Could you check a few things on this model? Use its own coordinates, in mm. A direction names the side the tool comes from. Give positions to 0.01 mm unless a question says otherwise; leave off trailing zeros. Order: outer loops, then holes, each group sorted by start corner. A loop starts at its lowest first (then second) coordinate and runs counter-clockwise, first axis right, second up. Notation, with made-up numbers: (89.25, -28.75) -> (134.25, -28.75) arc R13 ccw to (134.25, -14.75) -> close; hole circle Ø1 at (47.5, 83). An arc over 180 degrees is marked (long way). Write each question's results on one line, items separated by ' | '.
```python
from build123d import *

# Parameters (mm, degrees)
F1_DEPTH = 15


with BuildPart() as f1:
    # F0 (on Top) → F1 (new body)
    with BuildSketch(Plane.XY):
        Polygon((-70.779354, 10.755781), (-72.929354, 10.755781), (-72.929354, -4.244219), (-72.029354, -4.244219), (-68.829354, -4.244219), (-67.929354, -4.244219), (-67.929354, 10.755781), (-70.079354, 10.755781), align=None)
        Polygon((-71.429354, 14.255781), (-70.779354, 10.755781), (-70.079354, 10.755781), (-69.429354, 14.255781), align=None)
        Polygon((-72.029354, -4.244219), (-72.929354, -4.244219), (-72.929354, -7.944219), (-71.429354, -7.944219), align=None)
        Polygon((-67.929354, -4.244219), (-68.829354, -4.244219), (-69.429354, -7.944219), (-67.929354, -7.944219), align=None)
    extrude(amount=F1_DEPTH)


solid = f1.part
```
Q1. Suppose I cut it at B-B on y = -4.5. Please give me the cut outline in (x, z).
Here are the results:
outline: (-72.93, 0) -> (-71.99, 0) -> (-71.99, 15) -> (-72.93, 15) -> close; (-68.87, 0) -> (-67.93, 0) -> (-67.93, 15) -> (-68.87, 15) -> close
Q2. Thinking about a two-plate mould opening in X: for faces 6 (the flat face through (-71.11, 12.53, 7.4)), 7 (the flat face through (-69.125, -6.068, 7.395)), 8 (the flat face through (-69, 10.756, 7)), which applies, +X half, -X half, draft (parallel to the pull), parting line (faces both ways), or undercut?
Here are the results:
face 6: -X half | face 7: undercut | face 8: draft
Q3. Suppose I cut it at C-C on z = 13.5. Please give me the cut outline in (x, y).
Here are the results:
outline: (-72.93, -7.94) -> (-71.43, -7.94) -> (-72.03, -4.24) -> (-68.83, -4.24) -> (-69.43, -7.94) -> (-67.93, -7.94) -> (-67.93, 10.76) -> (-70.08, 10.76) -> (-69.43, 14.26) -> (-71.43, 14.26) -> (-70.78, 10.76) -> (-72.93, 10.76) -> close
Q4. Suppose I cut it at A-A on x = -69.05. Please give me the cut outline in (y, z).
Here are the results:
outline: (-7.94, 0) -> (-5.6, 0) -> (-5.6, 15) -> (-7.94, 15) -> close; (-4.24, 0) -> (10.76, 0) -> (10.76, 15) -> (-4.24, 15) -> close
Q5. I need wall thicknesses on line 1 along Y through (x, z) = (-68.7, 14); line 2 along Y through (x, z) = (-70.5, 2.25); line 3 along X through (y, z) = (-4.75, 4.25). Which ranges of each line are inside material? Lowest first, please.
Here are the results:
line 1: y = -7.94 to 10.76 | line 2: y = -4.24 to 14.26 | line 3: x = -72.93 to -71.95, -68.91 to -67.93
Q6. I'm going to push a flat-ended pin straight in: pin 1 Ø0.6 at (x, z) = (-72, 8) entering from +Y. Where does the tip first touch, or does it pass through?
Here are the results:
pin 1: stops at y = 10.76
Q7. For faces 1 (the flat face through (-71.725, -6.12, 7.395)), 2 (the flat face through (-70, 3, 15)), 3 (the flat face through (-69.76, 12.48, 7.4)), 4 (the flat face through (-72, 10.756, 7)), 5 (the flat face through (-67.929, 1, 7)), which set-ups out of +Z, -Z, +X, -X, +Y, -Y let a thin tool reach every point of the face, with its end or its side?
Here are the results:
face 1: +Z, -Z | face 2: +Z, +X, -X, +Y, -Y | face 3: +Z, -Z, +X | face 4: +Z, -Z, -X | face 5: +Z, -Z, +X, +Y, -Y
